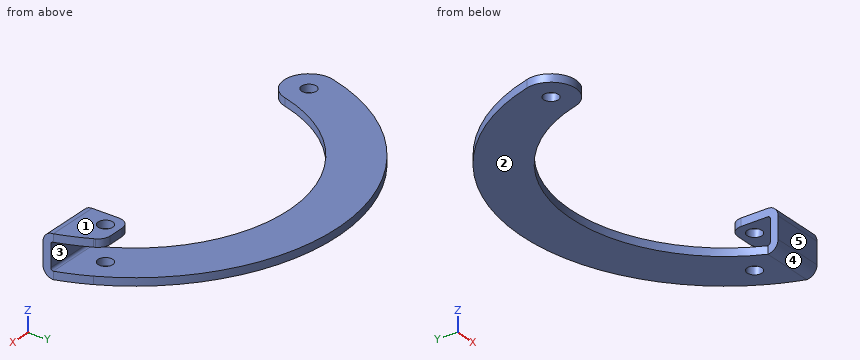
from build123d import *

# Parameters (mm, degrees)
BASE_FLANGE1_DEPTH           = 3.175
EDGE_FLANGE1_DEPTH           = 21.356037378
EDGE_FLANGE2_STRIP_W         = 14.7
EDGE_FLANGE2_STRIP_H         = 3.175
EDGE_FLANGE2_STRIP_CUT_DEPTH = 21.356037378
EDGE_FLANGE2_DEPTH           = 21.356037378
CUT_EXTRUDE1_DEPTH           = 160.658100285
CUT_EXTRUDE1_DEPTH_BACK      = 160.658100285
SKETCH12_R                   = 3
FILLET1_R                    = 5


# Sheet-metal steps are written as plain solids
with BuildPart() as part:
    # Sketch1 → Base-Flange1 (new body)
    with BuildSketch(Plane.XY):
        with BuildLine():
            Line((127.178904259, -0.503108866), (143.372130178, -0.503108866))
            Line((143.372130178, -0.503108866), (148.534941637, -0.503108866))
            ThreePointArc((148.534941637, -0.503108866), (146.210001092, 5.851436917), (143.372130178, 11.994082058))
            ThreePointArc((143.372130178, 11.994082058), (61.381820352, 56.404158269), (-9.649714749, -4.004341098))
            ThreePointArc((-9.649714749, -4.004341098), (-2.623548221, -16.277604067), (9.649714749, -9.251437539))
            ThreePointArc((9.649714749, -9.251437539), (65.321056088, 36.678957766), (127.178904259, -0.503108866))
        make_face()
    extrude(amount=-BASE_FLANGE1_DEPTH)

    # Edge-Flange1 section (across the edge) → Edge-Flange1 (add)
    with BuildSketch(Plane(origin=(127.178904259, -1.503108866, 0), x_dir=(0, 1, 0), z_dir=(1, 0, 0))):
        with BuildLine():
            Line((-3.175, 1), (-3.175, 10.825))
            Line((-3.175, 10.825), (0, 10.825))
            Line((0, 10.825), (0, 1))
            ThreePointArc((0, 1), (0.292893219, 0.292893219), (1, 0))
            Line((1, 0), (1, -3.175))
            ThreePointArc((1, -3.175), (-1.952170811, -1.952170811), (-3.175, 1))
        make_face()
    extrude(amount=EDGE_FLANGE1_DEPTH)

    # Edge-Flange2 strip (across the edge) → Edge-Flange2 strip cut (cut)
    with BuildSketch(Plane(origin=(127.178904259, -1.503108866, 10.825), x_dir=(0, 0, -1), z_dir=(1, 0, 0))):
        with Locations((-6.35, -1.5875)):
            Rectangle(EDGE_FLANGE2_STRIP_W, EDGE_FLANGE2_STRIP_H)
    extrude(amount=EDGE_FLANGE2_STRIP_CUT_DEPTH, mode=Mode.SUBTRACT)

    # Edge-Flange2 section (across the edge) → Edge-Flange2 (add)
    with BuildSketch(Plane(origin=(127.178904259, -1.503108866, 10.825), x_dir=(0, 0, -1), z_dir=(1, 0, 0))):
        with BuildLine():
            Line((-3.175, 1), (-3.175, 16.825))
            Line((-3.175, 16.825), (0, 16.825))
            Line((0, 16.825), (0, 1))
            ThreePointArc((0, 1), (0.292893219, 0.292893219), (1, 0))
            Line((1, 0), (1, -3.175))
            ThreePointArc((1, -3.175), (-1.952170811, -1.952170811), (-3.175, 1))
        make_face()
    extrude(amount=EDGE_FLANGE2_DEPTH)

    # Sketch12 → Cut-Extrude1 (cut, two sides: drawn at the far end of the back side and taken through both)
    with BuildSketch(Plane.XY.offset(-CUT_EXTRUDE1_DEPTH_BACK)):
        with Locations((133.372130178, 9.496891134)):
            Circle(SKETCH12_R)
        with Locations((0, -6.627889318)):
            Circle(SKETCH12_R)
        with BuildLine():
            Line((141.568166958, 15.321891134), (148.534941637, 15.321891134))
            Line((148.534941637, 15.321891134), (148.534941637, -0.503108866))
            ThreePointArc((148.534941637, -0.503108866), (146.210001092, 5.851436917), (143.372130178, 11.994082058))
            ThreePointArc((143.372130178, 11.994082058), (142.48923714, 13.66833427), (141.568166958, 15.321891134))
        make_face()
    extrude(amount=CUT_EXTRUDE1_DEPTH + CUT_EXTRUDE1_DEPTH_BACK, mode=Mode.SUBTRACT)

    # Fillet1
    fillet1_edges = [part.edges().sort_by_distance(p)[0] for p in [
        (127.178904259, 15.321891134, 12.4125),
        (141.568166958, 15.321891134, 12.4125),
    ]]
    fillet(fillet1_edges, radius=FILLET1_R)


solid = part.part
Build history of the part. All positions in model axes, mm. Face numbers are marked on the shaded views. A direction names the side the tool comes from. Round coordinates to 2 decimals unless told otherwise and drop trailing zeros. Loops run counter-clockwise (first coordinate to the right, second up) from the corner with the lowest first, then second, coordinate; pieces in that order, holes last. Notation, with made-up numbers: (83.5, 15) -> (121.5, 15) arc R11 ccw to (121.5, 23) -> close; hole circle Ø10 at (65, 8). An arc over 180 degrees is marked (long way). One line per item, written item: value. Start each with the question number.
Q1. Cut at D-D on x = 30. List the corners of the cut face in (y, z) (3 decimals), plus the area to 3 significant figures.
Q2. Cut at C-C on x = 0. List the corners of the cut face in (y, z) (3 decimals).
Q3. Cut at B-B on y = 34. List the corners of the cut face in (x, z) (3 decimals), plus the area to 3 significant figures.
Q4. 3-axis set-ups, long thin cutter, end or side, ignore diameter. For the marked faces 4 and 5: which of +Z, -Z, +X, -X, +Y, -Y reach the whole face in a straight line?
Q5. Cut at A-A on y = 4. List the corners of the cut face in (x, z) (3 decimals), plus the area to 3 significant figures.
Q6. Drop flat-ended pins along their axis: pin 1 Ø5 at (y, z) = (41, 1) entering from +X; pin 2 Ø1 at (x, z) = (135.5, 12.5) entering from +Y; pin 3 Ø2.5 at (x, z) = (136.5, 5) entering from +Y; pin 4 Ø17.5 at (x, y) = (133, 10.5) entering from -Z (3 decimals). Give the stop position or say it passes through.
Q7. Two-plate mould, pull along Z, no slides. Class the marked faces 1, 2 and 3: released by +Z, released by -Z, zero draft, split by the parting line, or undercut.
Q8. Probe line 1 along X through (y, z) = (-4, 6.5); line 2 along Z through (x, y) = (57, 37) (3 decimals); line 3 along Y through (x, z) = (41, -1). List the from-to ranges inside material, lowest first.
Computed:
1. outline: (22.408, -3.175) -> (46.528, -3.175) -> (46.528, 0) -> (22.408, 0) -> close
1. area: 76.6 mm²
2. outline: (-16.628, -3.175) -> (-9.628, -3.175) -> (-9.628, 0) -> (-16.628, 0) -> close; (-3.628, -3.175) -> (18.075, -3.175) -> (18.075, 0) -> (-3.628, 0) -> close
3. outline: (12.967, -3.175) -> (51.298, -3.175) -> (51.298, 0) -> (12.967, 0) -> close; (88.623, -3.175) -> (126.954, -3.175) -> (126.954, 0) -> (88.623, 0) -> close
3. area: 243 mm²
4. face 4: -Z, +X, -Y
4. face 5: +Z, -Z, +X, -X, -Y
5. outline: (-7.028, -3.175) -> (14.94, -3.175) -> (14.94, 0) -> (-7.028, 0) -> close; (124.981, -3.175) -> (146.949, -3.175) -> (146.949, 0) -> (124.981, 0) -> close; (127.179, 10.825) -> (146.949, 10.825) -> (146.949, 14) -> (127.179, 14) -> close
5. area: 202 mm²
6. pin 1: x = 121.58
6. pin 2: y = 15.32
6. pin 3: y = -1.5
6. pin 4: z = -3.175
7. face 1: released by +Z
7. face 2: released by -Z
7. face 3: undercut
8. line 1: 127.18 to 148.53
8. line 2: -3.175 to 0
8. line 3: 29.74 to 51.6
